from build123d import *

# Parameters (mm, degrees)
CROQUIS1_R               = 1.625
SALIENTE_EXTRUIR1_DEPTH  = 4
SALIENTE_EXTRUIR2_DEPTH  = 3.5
CORTAR_EXTRUIR1_START    = -98
CORTAR_EXTRUIR1_DEPTH    = 98
SALIENTE_EXTRUIR4_DEPTH  = 3.5
CROQUIS11_W              = 3.5
CROQUIS11_H              = 24.500023525
SALIENTE_EXTRUIR16_DEPTH = 43.75
CORTAR_EXTRUIR2_START    = -98
CROQUIS13_R              = 8
CORTAR_EXTRUIR2_DEPTH    = 98
SALIENTE_EXTRUIR17_DEPTH = 91
CROQUIS15_R              = 8
CORTAR_EXTRUIR3_DEPTH    = 70
SALIENTE_EXTRUIR18_DEPTH = 98
SALIENTE_EXTRUIR19_START = -3.5
SALIENTE_EXTRUIR19_DEPTH = 3.5
SALIENTE_EXTRUIR20_START = -3.5
SALIENTE_EXTRUIR20_DEPTH = 3.5
CROQUIS22_R              = 1.625
CROQUIS22_W              = 7.7
CROQUIS22_H              = 10
CORTAR_EXTRUIR4_DEPTH    = 4
SALIENTE_EXTRUIR21_DEPTH = 13
SALIENTE_EXTRUIR22_DEPTH = 13
SALIENTE_EXTRUIR23_DEPTH = 9.25
CORTAR_EXTRUIR5_START    = -12.474615
CORTAR_EXTRUIR5_DEPTH    = 12.474615
CROQUIS27_R              = 3.36
CORTAR_EXTRUIR6_DEPTH    = 1.8
CORTAR_EXTRUIR6_TAPER    = 44


with BuildPart() as part:
    # Croquis1 → Saliente-Extruir1 (new body)
    with BuildSketch(Plane.XY):
        Polygon((99, -28), (99, -98), (1, -98), (1, -28), (22, -28), (22, 0), (78, 0), (78, -28), align=None)
        with Locations((29, -3.05)):
            Circle(CROQUIS1_R, mode=Mode.SUBTRACT)
        with Locations((29, -26.05)):
            Circle(CROQUIS1_R, mode=Mode.SUBTRACT)
        with Locations((71, -26.05)):
            Circle(CROQUIS1_R, mode=Mode.SUBTRACT)
        with Locations((71, -3.05)):
            Circle(CROQUIS1_R, mode=Mode.SUBTRACT)
    extrude(amount=SALIENTE_EXTRUIR1_DEPTH)

    # Croquis3 → Saliente-Extruir2 (add)
    with BuildSketch(Plane.ZY.offset(-1)):
        Polygon((4, -74.869484932), (3.981861285, -95.48724368), (5.706893625, -94.286253678), (28.5, -87.835533437), (28.5, -74.835533437), align=None)
    extrude(amount=-SALIENTE_EXTRUIR2_DEPTH)

    # Croquis4 → Cortar-Extruir1 (cut)
    with BuildSketch(Plane.ZY.offset(-1).offset(CORTAR_EXTRUIR1_START)):
        Polygon((4, -98), (0.372683932, -98), (4, -95.47461527), align=None)
    extrude(amount=CORTAR_EXTRUIR1_DEPTH, mode=Mode.SUBTRACT)

    # Croquis6 → Saliente-Extruir4 (add)
    with BuildSketch(Plane(origin=(99, 0, 0), x_dir=(0, 0, -1), z_dir=(1, 0, 0))):
        Polygon((-4, -95.47461527), (-5.706893625, -94.286253678), (-28.5, -87.835533437), (-28.5, -74.835533437), (-4, -74.869484932), align=None)
    extrude(amount=-SALIENTE_EXTRUIR4_DEPTH)

    # Croquis11 → Saliente-Extruir16 (add)
    with BuildSketch(Plane(origin=(0, -74.874884245, 0.103759765), x_dir=(1, 0, 0), z_dir=(0, 0.99999904, -0.001385774))):
        with Locations((97.25, -16.146255738)):
            Rectangle(CROQUIS11_W, CROQUIS11_H)
        with Locations((2.75, -16.146255738)):
            Rectangle(CROQUIS11_W, CROQUIS11_H)
    extrude(amount=SALIENTE_EXTRUIR16_DEPTH)

    # Croquis13 → Cortar-Extruir2 (cut)
    with BuildSketch(Plane.ZY.offset(-1).offset(CORTAR_EXTRUIR2_START)):
        with Locations((19.5, -42.25)):
            Circle(CROQUIS13_R)
        with Locations((19.5, -66.75)):
            Circle(CROQUIS13_R)
    extrude(amount=CORTAR_EXTRUIR2_DEPTH, mode=Mode.SUBTRACT)

    # Croquis14 → Saliente-Extruir17 (add)
    with BuildSketch(Plane.ZY.offset(-95.5)):
        Polygon((28.5, -87.835533437), (5.706893625, -94.286253678), (4, -95.47461527), (4, -88.47461527), (28.5, -83.835533437), align=None)
    extrude(amount=SALIENTE_EXTRUIR17_DEPTH)

    # Croquis15 → Cortar-Extruir3 (cut)
    with BuildSketch(Plane.XZ.offset(98)):
        with Locations((37.75, 19.5)):
            Circle(CROQUIS15_R)
        with Locations((62.25, 19.5)):
            Circle(CROQUIS15_R)
    extrude(amount=-CORTAR_EXTRUIR3_DEPTH, mode=Mode.SUBTRACT)

    # Croquis18 → Saliente-Extruir18 (add)
    with BuildSketch(Plane(origin=(99, 0, 0), x_dir=(0, 0, -1), z_dir=(1, 0, 0))):
        Polygon((-28.5, -87.835533437), (-33.311039019, -86.473952165), (-33.311039019, -82.473952165), (-28.5, -83.835533437), align=None)
    extrude(amount=-SALIENTE_EXTRUIR18_DEPTH)

    # Croquis19 → Saliente-Extruir19 (add)
    with BuildSketch(Plane(origin=(99, 0, 0), x_dir=(0, 0, -1), z_dir=(1, 0, 0)).offset(SALIENTE_EXTRUIR19_START)):
        Polygon((-28.5, -83.835533437), (-33.311039019, -82.473952165), (-33.311039019, -31.085575445), (-28.439372389, -31.085575445), (-28.5, -74.835533437), align=None)
    extrude(amount=SALIENTE_EXTRUIR19_DEPTH)

    # Croquis20 → Saliente-Extruir20 (add)
    with BuildSketch(Plane.ZY.offset(-1).offset(SALIENTE_EXTRUIR20_START)):
        Polygon((28.439372389, -31.085575445), (33.311039019, -31.085575445), (33.311039019, -82.473952165), (28.5, -83.835533437), (28.5, -74.835533437), align=None)
    extrude(amount=SALIENTE_EXTRUIR20_DEPTH)

    # Croquis22 → Cortar-Extruir4 (cut)
    with BuildSketch(Plane.XY.offset(4)):
        with Locations((88.362832, -80.438630677)):
            Circle(CROQUIS22_R)
        with Locations((11.637168, -80.438630677)):
            Circle(CROQUIS22_R)
        with Locations((82.35, -80.438630677)):
            Rectangle(CROQUIS22_W, CROQUIS22_H)
        with Locations((17.65, -80.438630677)):
            Rectangle(CROQUIS22_W, CROQUIS22_H)
    extrude(amount=-CORTAR_EXTRUIR4_DEPTH, mode=Mode.SUBTRACT)

    # Croquis23 → Saliente-Extruir21 (add)
    with BuildSketch(Plane(origin=(4.5, 0, 0), x_dir=(0, 0, -1), z_dir=(1, 0, 0))):
        with BuildLine():
            Line((-13.255002002, -71.75), (-4, -71.75))
            Line((-4, -71.75), (-4, -61.75))
            Line((-4, -61.75), (-13.255002002, -61.75))
            ThreePointArc((-13.255002002, -61.75), (-11.5, -66.75), (-13.255002002, -71.75))
        make_face()
        with BuildLine():
            Line((-4, -47.25), (-13.255002002, -47.25))
            ThreePointArc((-13.255002002, -47.25), (-11.5, -42.25), (-13.255002002, -37.25))
            Line((-13.255002002, -37.25), (-4, -37.25))
            Line((-4, -37.25), (-4, -47.25))
        make_face()
    extrude(amount=SALIENTE_EXTRUIR21_DEPTH)

    # Croquis24 → Saliente-Extruir22 (add)
    with BuildSketch(Plane.ZY.offset(-95.5)):
        with BuildLine():
            Line((13.255002002, -37.25), (4, -37.25))
            Line((4, -37.25), (4, -47.25))
            Line((4, -47.25), (13.255002002, -47.25))
            ThreePointArc((13.255002002, -47.25), (11.5, -42.25), (13.255002002, -37.25))
        make_face()
        with BuildLine():
            Line((13.255002002, -61.75), (4, -61.75))
            Line((4, -61.75), (4, -71.75))
            Line((4, -71.75), (13.255002002, -71.75))
            ThreePointArc((13.255002002, -71.75), (11.5, -66.75), (13.255002002, -61.75))
        make_face()
    extrude(amount=SALIENTE_EXTRUIR22_DEPTH)

    # Croquis25 → Saliente-Extruir23 (add)
    with BuildSketch(Plane.XY.offset(4)):
        Polygon((37.75, -88.47461527), (42.75, -88.47461527), (42.75, -76), (32.75, -76), (32.75, -88.47461527), align=None)
        Polygon((62.25, -88.47461527), (67.25, -88.47461527), (67.25, -76), (57.25, -76), (57.25, -88.47461527), align=None)
    extrude(amount=SALIENTE_EXTRUIR23_DEPTH)

    # Croquis26 → Cortar-Extruir5 (cut)
    with BuildSketch(Plane.XZ.offset(88.47461527).offset(CORTAR_EXTRUIR5_START)):
        with BuildLine():
            Line((57.256253911, 13.25), (67.243746089, 13.25))
            ThreePointArc((67.243746089, 13.25), (62.25, 11.5), (57.256253911, 13.25))
        make_face()
        with BuildLine():
            Line((32.756253911, 13.25), (42.743746089, 13.25))
            ThreePointArc((42.743746089, 13.25), (37.75, 11.5), (32.756253911, 13.25))
        make_face()
    extrude(amount=CORTAR_EXTRUIR5_DEPTH, mode=Mode.SUBTRACT)

    # Croquis27 → Cortar-Extruir6 (cut)
    with BuildSketch(Plane(origin=(0, 0, 0), x_dir=(-1, 0, 0), z_dir=(0, 0, -1))):
        with Locations((-29, -26.05)):
            Circle(CROQUIS27_R)
        with Locations((-71, -26.05)):
            Circle(CROQUIS27_R)
        with Locations((-71, -3.05)):
            Circle(CROQUIS27_R)
        with Locations((-29, -3.05)):
            Circle(CROQUIS27_R)
        with Locations((-11.637168, -80.438630677)):
            Circle(CROQUIS27_R)
        with Locations((-88.362832, -80.438630677)):
            Circle(CROQUIS27_R)
    extrude(amount=-CORTAR_EXTRUIR6_DEPTH, taper=CORTAR_EXTRUIR6_TAPER, mode=Mode.SUBTRACT)


solid = part.part
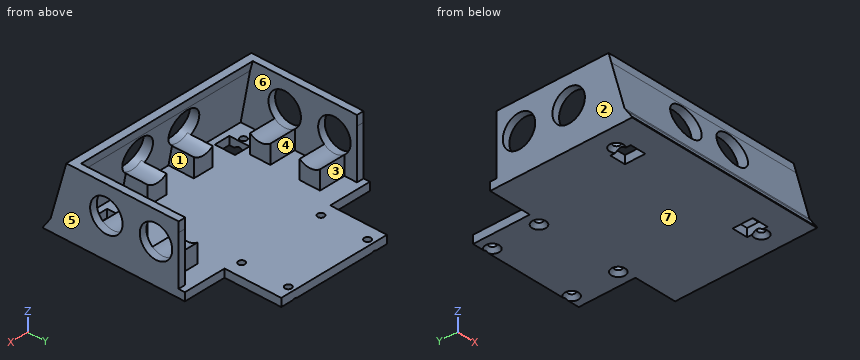
Work out the finished part from the listing and answer in its coordinate system (mm). Face numbers are marked on the shaded views. A direction names the side the tool comes from. Round coordinates to 2 decimals unless told otherwise and drop trailing zeros. Loops run counter-clockwise (first coordinate to the right, second up) from the corner with the lowest first, then second, coordinate; pieces in that order, holes last. Notation, with made-up numbers: M 79,-40 L 110,-40 A14 cw 110,-29 Z; hole C -38.5,45 d9. An arc over 180 degrees is marked long. One line per question, with ' | ' between items. Start each with the question number.
(1) Find the intervals of material crossed by line 1 (X direction, y = -43.5, z = 28); line 2 (X direction, y = -26.05, z = 3.5) (3 decimals); line 3 (Y direction, x = 71, z = 2.9) (3 decimals), in increasing order.
(2) Flat-ended cylindrical pins translate along their axes: pin 1 Ø2 at (y, z) = (-19.5, 1) entering from -X; pin 2 Ø6 at (x, z) = (17.5, 21.5) entering from -Y; pin 3 Ø3 at (x, z) = (12, 1.5) entering from +Y. Find the tip coordinate at first contact, or state that the pin passes through.
(3) A cutting plane is placed at D-D on y = -40. Write down the section's boundary in (x, z), plus the area to 3 significant figures.
(4) A tool of negligible diameter and unlimited length cuts with its end or side. For the marked faces 1, 2 and 3, from which of +Z, -Z, +X, -X, +Y, -Y can it reach the whole face along a straight path? Write none if from no direction.
(5) A cutting plane is placed at A-A on y = -66.75. Write down the section's boundary in (x, z).
(6) A cutting plane is placed at C-C on z = 19.5. Give the number of separate pieces and of enclosed holes in the cut face, plus the area to 3 significant figures.
(7) For a pull along X with two mould halves and no side action, classify the marked faces 4, 5, 6 and 7 as released by +X, released by -X, zero draft, split by the parting line, or undercut.
(8) A cutting plane is placed at B-B on x = 39. Write down the section's boundary in (y, z).
Geometry check:
1) line 1: x = 1 to 4.5, 95.5 to 99 | line 2: x = 22 to 27.375, 30.625 to 69.375, 72.625 to 78 | line 3: y = -96.24 to -27.675, -24.425 to -4.675, -1.425 to 0
2) pin 1: stops at x = 22 | pin 2: stops at y = -90.67 | pin 3: stops at y = -28
3) outline: M 1,0 L 99,0 L 99,11.82 L 82.5,11.82 L 82.5,4 L 17.5,4 L 17.5,11.82 L 1,11.82 Z; M 1,27.18 L 4.5,27.18 L 4.5,33.31 L 1,33.31 Z; M 95.5,27.18 L 99,27.18 L 99,33.31 L 95.5,33.31 Z | area: 693 mm²
4) face 1: +Y | face 2: +Z, -Z, -X, +Y, -Y | face 3: +Z, +Y
5) outline: M 1,0 L 99,0 L 99,11.5 L 82.5,11.5 L 82.5,4 L 17.5,4 L 17.5,11.5 L 1,11.5 Z; M 1,27.5 L 4.5,27.5 L 4.5,33.31 L 1,33.31 Z; M 95.5,27.5 L 99,27.5 L 99,33.31 L 95.5,33.31 Z
6) separate pieces: 7 | enclosed holes: 0 | area: 477 mm²
7) face 4: undercut | face 5: released by +X | face 6: undercut | face 7: zero draft
8) outline: M -98,0 L 0,0 L 0,4 L -76,4 L -76,11.6 L -92.62,11.6 L -94.29,5.71 L -98,0.37 Z; M -88.15,27.4 L -84.04,27.4 L -83.84,28.5 L -82.47,33.31 L -86.47,33.31 Z
